Read the model definition and answer for the solid it produces. Units are mm, in the model's axes. Face numbers are marked on the shaded views. A direction names the side the tool comes from. Give positions to 0.01 mm unless a question says otherwise; leave off trailing zeros. Loops run counter-clockwise (first coordinate to the right, second up) from the corner with the lowest first, then second, coordinate; pieces in that order, holes last.
(1) Straight lines are drawn through the part: probe 1 along X at (y, z) = (0.85, -2.54); probe 2 along Y at (x, z) = (16.5, 1); probe 3 along X at (y, z) = (1, -2). For each, find the intervals that lie inside material, in ascending order.
(2) Find section D-D, the plane x = 11. Write down the section's boundary in (y, z).
(3) Determine the mould class of the marked faces 5, 6, 7 and 8 for opening direction X: pulls with the +X half, pulls with the -X half, needs draft (parallel to the pull), parting line crosses it, or undercut.
(4) Find section C-C, the plane z = -2.54. Write down the section's boundary in (x, y).
(5) Which of the six approach directions +Z, -Z, +X, -X, +Y, -Y give full straight-line access (tool end or side, diameter ignored) to the marked faces 1, 2, 3 and 4?
(6) Each of these flat-tipped pins is pushed along its axis until it touches: P1, Ø3, axis at y = 3.5, z = 4.5, coming from the +X side; P2, Ø0.6, axis at x = -11.5, y = 2, coming from the +Z side; P3, Ø5, axis at x = -2.5, z = -1, coming from the +Y side; P4, Ø1.7, axis at x = 19.05, z = -2.54, coming from the +Y side. Where does it stop, or does it pass through?
(7) Find section A-A, the plane x = -19.05. Write down the section's boundary in (y, z).
(8) Find section B-B, the plane y = 5. Write down the section's boundary in (x, z), then the cut area to 3 significant figures.
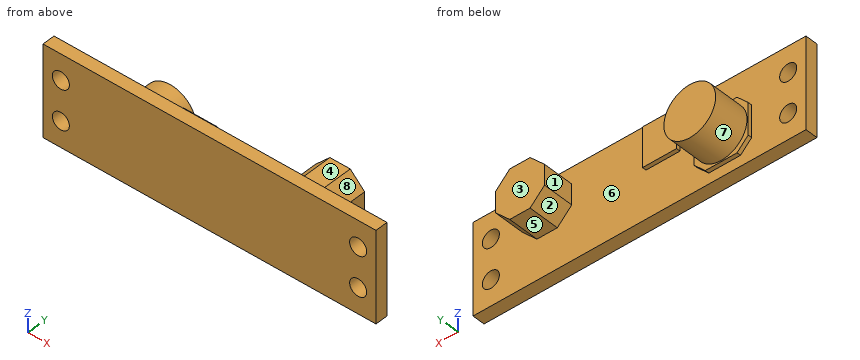
```python
from build123d import *

# Parameters (mm, degrees)
SKETCH1_W           = 42.672
SKETCH1_H           = 11.684
SKETCH1_R           = 1.0922
BOSS_EXTRUDE1_DEPTH = 1.6002
SKETCH2_W           = 4.360829253
SKETCH2_H           = 5.074241287
BOSS_EXTRUDE2_DEPTH = 0.508
BOSS_EXTRUDE3_DEPTH = 0.508
SKETCH4_R           = 3.318325067
BOSS_EXTRUDE4_DEPTH = 4.572
BOSS_EXTRUDE5_DEPTH = 3.96875


with BuildPart() as part:
    # Sketch1 → Boss-Extrude1 (new body)
    with BuildSketch(Plane(origin=(0, 0, 0), x_dir=(1, 0, 0), z_dir=(0, 1, 0))):
        Rectangle(SKETCH1_W, SKETCH1_H)
        with Locations(Location((-19.05, 2.54, 0), (0, 0, 270))):
            Circle(SKETCH1_R, mode=Mode.SUBTRACT)
        with Locations(Location((-19.05, -2.54, 0), (0, 0, 270))):
            Circle(SKETCH1_R, mode=Mode.SUBTRACT)
        with Locations(Location((19.05, 2.54, 0), (0, 0, 270))):
            Circle(SKETCH1_R, mode=Mode.SUBTRACT)
        with Locations(Location((19.05, -2.54, 0), (0, 0, 270))):
            Circle(SKETCH1_R, mode=Mode.SUBTRACT)
    extrude(amount=BOSS_EXTRUDE1_DEPTH)

    # Sketch2 → Boss-Extrude2 (add)
    with BuildSketch(Plane(origin=(0, 1.6002, 0), x_dir=(1, 0, 0), z_dir=(0, 1, 0))):
        with Locations((-3.010313867, -2.820245611)):
            Rectangle(SKETCH2_W, SKETCH2_H)
    extrude(amount=BOSS_EXTRUDE2_DEPTH)

    # Sketch3 → Boss-Extrude3 (add)
    with BuildSketch(Plane(origin=(0, 1.6002, 0), x_dir=(1, 0, 0), z_dir=(0, 1, 0))):
        Polygon((-7.440948477, -1.028779312), (-7.440948477, 3.035220688), (-8.877789457, 4.472061667), (-12.941789457, 4.472061667), (-14.378630436, 3.035220688), (-14.378630436, -1.028779312), (-12.941789457, -2.465620292), (-8.877789457, -2.465620292), align=None)
    extrude(amount=BOSS_EXTRUDE3_DEPTH)

    # Sketch4 → Boss-Extrude4 (add)
    with BuildSketch(Plane(origin=(0, 2.1082, 0), x_dir=(1, 0, 0), z_dir=(0, 1, 0))):
        with Locations(Location((-10.909789457, 1.003220688, 0), (0, 0, 90))):
            Circle(SKETCH4_R)
    extrude(amount=BOSS_EXTRUDE4_DEPTH)

    # Sketch5 → Boss-Extrude5 (add)
    with BuildSketch(Plane(origin=(0, 1.6002, 0), x_dir=(1, 0, 0), z_dir=(0, 1, 0))):
        Polygon((14.986, -3.741894505), (14.986, -1.131751289), (13.140350032, 0.71389868), (10.530206815, 0.71389868), (8.684556847, -1.131751289), (8.684556847, -3.741894505), (10.530206815, -5.587544473), (13.140350032, -5.587544473), align=None)
    extrude(amount=BOSS_EXTRUDE5_DEPTH)


solid = part.part
```
Entries:
1. probe 1: x = -21.34 to -20.14, -17.96 to 17.96, 20.14 to 21.34
1. probe 2: y = 0 to 1.6
1. probe 3: x = -21.34 to -20, -18.1 to 18.1, 20 to 21.34
2. outline: (0, -5.84) - (1.6, -5.84) - (1.6, -0.71) - (5.57, -0.71) - (5.57, 5.59) - (1.6, 5.59) - (1.6, 5.84) - (0, 5.84) - close
3. face 5: needs draft
3. face 6: undercut
3. face 7: undercut
3. face 8: pulls with the +X half
4. outline: (-21.34, 0) - (-20.14, 0) - (-20.14, 1.6) - (-21.34, 1.6) - close; (-17.96, 0) - (17.96, 0) - (17.96, 1.6) - (-7.44, 1.6) - (-7.44, 2.11) - (-7.97, 2.11) - (-7.97, 6.68) - (-13.85, 6.68) - (-13.85, 2.11) - (-14.38, 2.11) - (-14.38, 1.6) - (-17.96, 1.6) - close; (20.14, 0) - (21.34, 0) - (21.34, 1.6) - (20.14, 1.6) - close
5. face 1: +Z, -Z, +Y
5. face 2: -Z, +Y
5. face 3: +Z, -Z, +X, +Y
5. face 4: +Z, +X, -X, +Y
6. P1: stops at x = 14.99
6. P2: stops at z = 2.47
6. P3: stops at y = 2.11
6. P4: passes through
7. outline: (0, -5.84) - (1.6, -5.84) - (1.6, -3.63) - (0, -3.63) - close; (0, -1.45) - (1.6, -1.45) - (1.6, 1.45) - (0, 1.45) - close; (0, 3.63) - (1.6, 3.63) - (1.6, 5.84) - (0, 5.84) - close
8. outline: circle Ø6.64 at (-10.91, -1); (8.68, 1.13) - (10.53, -0.71) - (13.14, -0.71) - (14.99, 1.13) - (14.99, 3.74) - (13.14, 5.59) - (10.53, 5.59) - (8.68, 3.74) - close
8. area: 67.5 mm2
